Here's the drawing with two shaded views (mm, measured from the low corner). I have some questions. A direction names the side the tool comes from. Coordinates: 2 decimals unless noted, no trailing zeros. Order: outer loops, then holes, each group sorted by start corner. A loop starts at its lowest first (then second) coordinate and runs counter-clockwise, first axis right, second up. Notation, with made-up numbers: M 39.5,-24 L 74.5,-24 A23 ccw 74.5,-9 Z; hole C 41.5,38 d10. An arc over 180 degrees is marked long. Put each result on its own line as item: value. Start each with the question number.
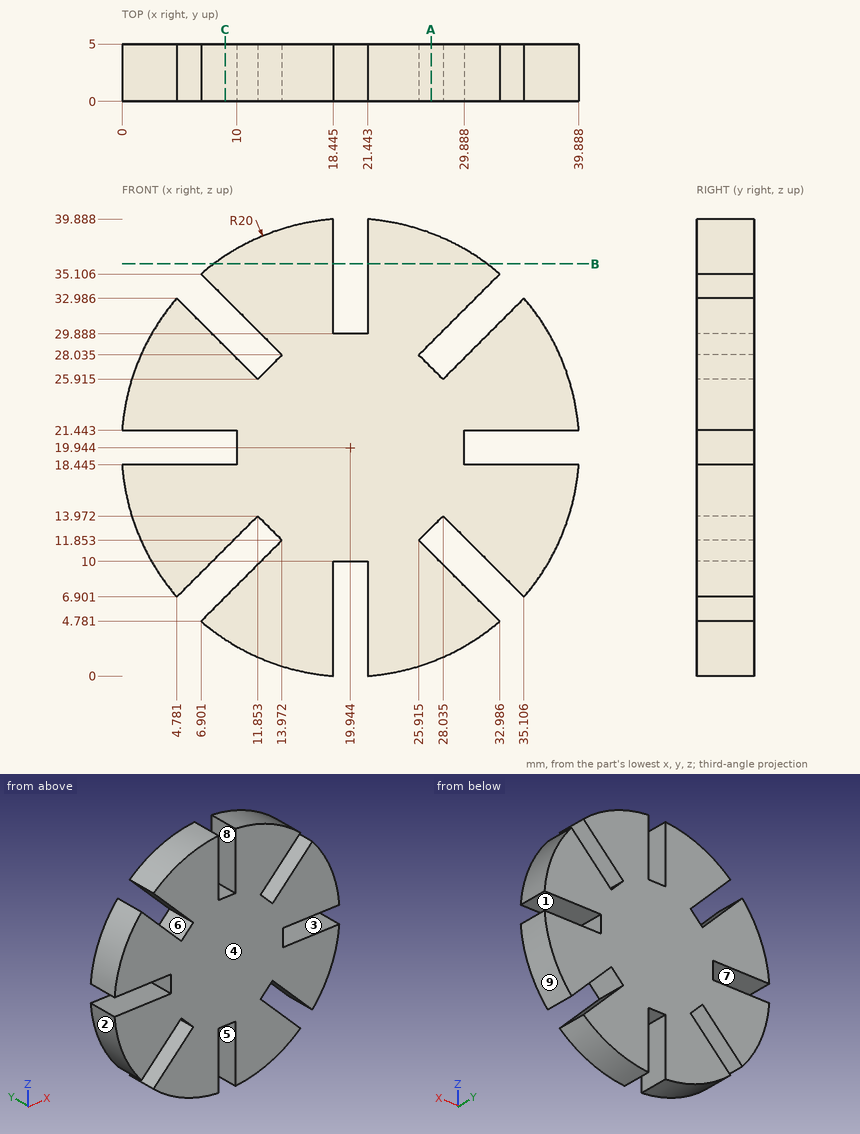
Item 1: For the marked faces 5, 6, 7, 8 and 9, which set-ups out of +Z, -Z, +X, -X, +Y, -Y let a thin tool reach every point of the face, with its end or its side?
Item 2: If we section it at C-C on x = 9: Write out the boundary of the cut face in (y, z) (1 decimal).
Item 3: If we mould it in two halves opening along Z, with no side actions, what happens to the marked faces 1, 2, 3 and 4? For each: released by +Z, released by -Z, zero draft, split by the parting line, or undercut.
Item 4: If we section it at A-A on x = 27: Write out the boundary of the cut face in (y, z).
Item 5: If we section it at B-B on z = 36: Write out the boundary of the cut face in (x, y) (1 decimal).
Item 6: I need wall thicknesses on probe 1 along X at (y, z) = (3.9, 31) (1 decimal); probe 2 along Z at (x, y) = (28.5, 2.3) (1 decimal); probe 3 along X at (y, z) = (1.05, 8.5) (1 decimal). Which ranges of each line are inside material? Lowest first, please.
Item 7: For pin 1 Ø0.9 at (x, y) = (20, 2.5) entering from +Z; pin 2 Ø2.5 at (y, z) = (2, 7) entering from -X; pin 3 Ø1.5 at (x, y) = (34.5, 3.5) entering from -Z, each with a flat end and sliding along its axis, tell me the tip position at first contact or that it passes through.
Geometry check:
1. face 5: -Z, +Y, -Y
1. face 6: +Y, -Y
1. face 7: -X, +Y, -Y
1. face 8: +Z, +Y, -Y
1. face 9: -Z, +X, +Y, -Y
2. outline: M 0,3.2 L 5,3.2 L 5,6.9 L 0,6.9 Z; M 0,11.1 L 5,11.1 L 5,18.4 L 0,18.4 Z; M 0,21.4 L 5,21.4 L 5,28.8 L 0,28.8 Z; M 0,33 L 5,33 L 5,36.7 L 0,36.7 Z
3. face 1: undercut
3. face 2: released by -Z
3. face 3: undercut
3. face 4: zero draft
4. outline: M 0,1.23 L 5,1.23 L 5,10.77 L 0,10.77 Z; M 0,12.94 L 5,12.94 L 5,26.95 L 0,26.95 Z; M 0,29.12 L 5,29.12 L 5,38.66 L 0,38.66 Z
5. outline: M 8,0 L 18.4,0 L 18.4,5 L 8,5 Z; M 21.4,0 L 31.9,0 L 31.9,5 L 21.4,5 Z
6. probe 1: x = 3.3 to 6.8, 11 to 18.4, 21.4 to 28.9, 33.1 to 36.6
6. probe 2: z = 1.9 to 9.3, 13.5 to 26.4, 30.6 to 38
6. probe 3: x = 3.5 to 6.4, 10.6 to 18.4, 21.4 to 29.3, 33.5 to 36.3
7. pin 1: stops at z = 29.89
7. pin 2: stops at x = 3.72
7. pin 3: stops at z = 6.9
